```python
from build123d import *

# Parameters (mm, degrees)
F0_R     = 40
F0_R_2   = 1.5
F0_R_3   = 25
F1_DEPTH = 3


with BuildPart() as f1:
    # F0 (on Top) → F1 (new body)
    with BuildSketch(Plane.XY):
        Circle(F0_R)
        Polygon((1.419746, -28.955333), (-0.080254, -28.955333), (-1.580254, -28.955333), (-1.580254, -27.955333), (1.419746, -27.955333), align=None, mode=Mode.SUBTRACT)
        Polygon((-29.014116, -1.51), (-29.014116, -0.01), (-29.014116, 1.49), (-28.014116, 1.49), (-28.014116, -1.51), align=None, mode=Mode.SUBTRACT)
        Polygon((-1.5, -35.965448), (0, -35.965448), (1.5, -35.965448), (1.5, -36.965448), (-1.5, -36.965448), align=None, mode=Mode.SUBTRACT)
        with Locations((0, -32.5)):
            Circle(F0_R_2, mode=Mode.SUBTRACT)
        Polygon((28.958499, 1.457314), (28.958499, -0.042686), (28.958499, -1.542686), (27.958499, -1.542686), (27.958499, 1.457314), align=None, mode=Mode.SUBTRACT)
        Polygon((-36.050154, 1.510031), (-36.050154, 0.010031), (-36.050154, -1.489969), (-37.050154, -1.489969), (-37.050154, 1.510031), align=None, mode=Mode.SUBTRACT)
        with Locations((-32.5, 0)):
            Circle(F0_R_2, mode=Mode.SUBTRACT)
        Circle(F0_R_3, mode=Mode.SUBTRACT)
        with Locations((32.5, 0)):
            Circle(F0_R_2, mode=Mode.SUBTRACT)
        Polygon((36.007276, -1.479468), (36.007276, 0.020532), (36.007276, 1.520532), (37.007276, 1.520532), (37.007276, -1.479468), align=None, mode=Mode.SUBTRACT)
        Polygon((-1.5, 29), (0, 29), (1.5, 29), (1.5, 28), (-1.5, 28), align=None, mode=Mode.SUBTRACT)
        with Locations((0, 32.5)):
            Circle(F0_R_2, mode=Mode.SUBTRACT)
        Polygon((1.5, 36), (0, 36), (-1.5, 36), (-1.5, 37), (1.5, 37), align=None, mode=Mode.SUBTRACT)
    extrude(amount=F1_DEPTH)


solid = f1.part
```
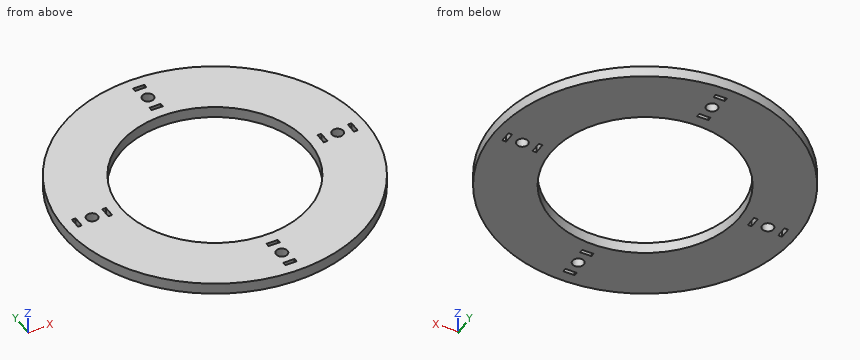
Check sheet for the modelled part. Datum: model origin and axes. Units: mm. Give positions to 0.01 mm unless a question says otherwise; leave off trailing zeros. Loops run counter-clockwise (first coordinate to the right, second up) from the corner with the lowest first, then second, coordinate; pieces in that order, holes last. Notation, with made-up numbers: M 51,-36.75 L 59,-36.75 A13 cw 59,-19.75 Z; hole C -14,-25.75 d11. An arc over 180 degrees is marked long. Answer in a Markdown table with one row per item.
1) Cross-section at A-A (y = 0). Count the separate pieces of the cut face and the enclosed holes in it, plus the area to 3 significant figures.
Solutions:
| item | result |
|---|---|
| separate pieces | 8 |
| enclosed holes | 0 |
| area | 60.0 mm^2 |
2) Cross-section at C-C (y = 32.5). Enter the section's corners in (x, z), plus the area to 3 significant figures.
Solutions:
| item | result |
|---|---|
| outline | M -23.32,0 L -1.5,0 L -1.5,3 L -23.32,3 Z; M 1.5,0 L 23.32,0 L 23.32,3 L 1.5,3 Z |
| area | 131 mm^2 |
3) Depth check by flat-ended pin: pin 1 (1 mm diameter, centred on y = -20.5, z = 1.5, fed in from -X); pin 2 (1.5 mm diameter, centred on x = 0, z = 1, fed in from -Y); pin 3 (5 mm diameter, centred on x = 0, y = 32.5, fed in from -Z); pin 4 (0.8 mm diameter, centred on x = 36.5, z = 2, fed in from -Y). Enter the tip coordinate at first touch or a pass-through.
Solutions:
| item | result |
|---|---|
| pin 1 | stops at x = -34.64 |
| pin 2 | stops at y = -40 |
| pin 3 | stops at z = 0 |
| pin 4 | stops at y = -17.23 |
4) Cross-section at B-B (x = -12). Enter the section's corners in (y, z), plus the area to 3 significant figures.
Solutions:
| item | result |
|---|---|
| outline | M -38.16,0 L -21.93,0 L -21.93,3 L -38.16,3 Z; M 21.93,0 L 38.16,0 L 38.16,3 L 21.93,3 Z |
| area | 97.4 mm^2 |
5) Thickness scan on line 1 (Y direction, x = 32.5, z = 1.9); line 2 (X direction, y = 32, z = 1.1); line 3 (Y direction, x = -4, z = 2.5). Record the ranges inside material, lowest first.
Solutions:
| item | result |
|---|---|
| line 1 | y = -23.32 to -1.5, 1.5 to 23.32 |
| line 2 | x = -24 to -1.41, 1.41 to 24 |
| line 3 | y = -39.8 to -24.68, 24.68 to 39.8 |
